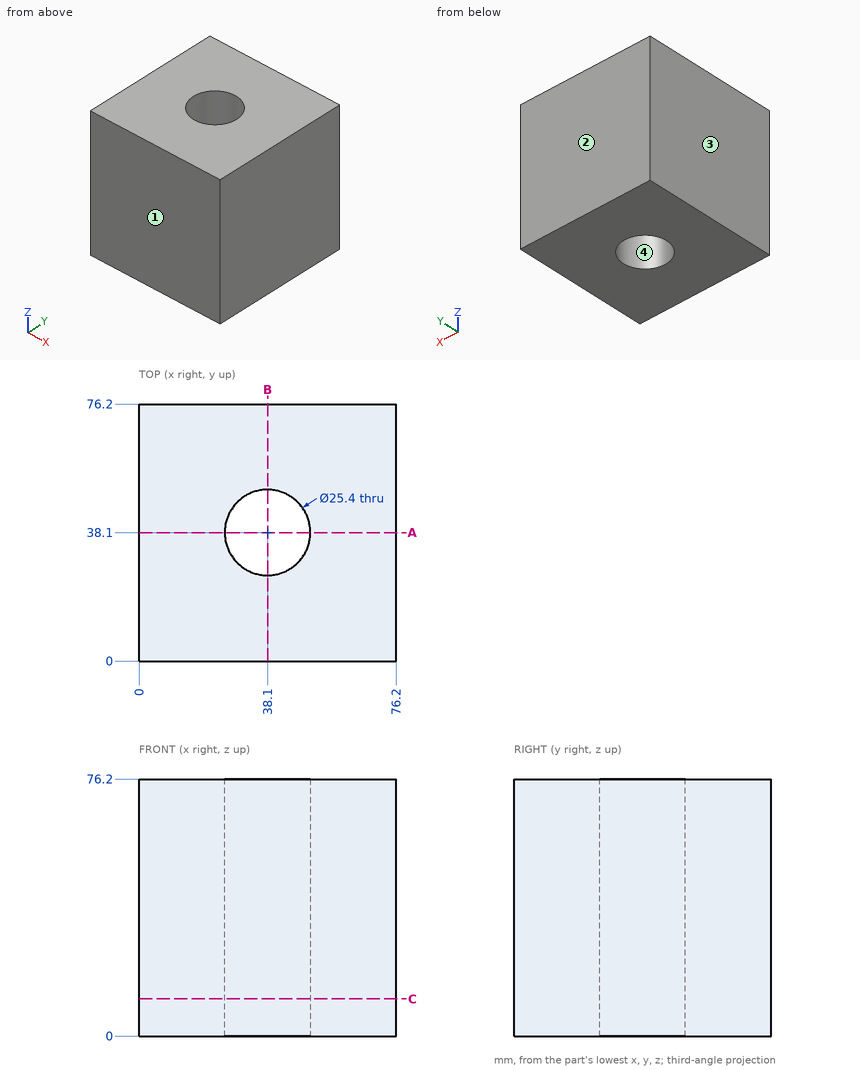
Geometry: see drawing. Coordinates: mm, zero at the bounding-box minimum. Coordinates: 2 decimals unless noted, no trailing zeros. Loops run counter-clockwise (first coordinate to the right, second up) from the corner with the lowest first, then second, coordinate; pieces in that order, holes last.
Q1. Contact query for a flat-ended pin moving along its axis: pin 1 (15 mm diameter, centred on x = 38.1, y = 38.1, fed in from -Z). Output: stop coordinate, or through.
Q2. Cut plane A-A (y = 38.1). Output: boundary loops of the cut face in (x, z), then the cut area to 3 significant figures.
Q3. Draft query along Y for the marked faces 1, 2, 3 and 4. Return one class per face: +Y half, -Y half, draft (parallel to the pull), parting line (faces both ways), or undercut.
Q4. Material intervals for line 1 (Y direction, x = 38, z = 51); line 2 (X direction, y = 42, z = 70.5), sorted ascending.
Q5. Cut plane C-C (z = 11). Output: boundary loops of the cut face in (x, y), then the cut area to 3 significant figures.
Working result:
1. pin 1: passes through
2. outline: (0, 0) - (25.4, 0) - (25.4, 76.2) - (0, 76.2) - close; (50.8, 0) - (76.2, 0) - (76.2, 76.2) - (50.8, 76.2) - close
2. area: 3,870 mm2
3. face 1: -Y half
3. face 2: +Y half
3. face 3: draft
3. face 4: undercut
4. line 1: y = 0 to 25.4, 50.8 to 76.2
4. line 2: x = 0 to 26.01, 50.19 to 76.2
5. outline: (0, 0) - (76.2, 0) - (76.2, 76.2) - (0, 76.2) - close; hole circle Ø25.4 at (38.1, 38.1)
5. area: 5,300 mm2
